Source: CAD feature listing. Evaluate the final solid. Frame: model axes, mm. Give positions to 0.01 mm unless a question says otherwise; leave off trailing zeros. Order: outer loops, then holes, each group sorted by start corner. A loop starts at its lowest first (then second) coordinate and runs counter-clockwise, first axis right, second up. Notation, with made-up numbers: M -13.5,-31 L 16.5,-31 A17 cw 16.5,-6 Z; hole C 16.25,70.25 d6. An arc over 180 degrees is marked long. Answer in a Markdown table with one row per item. Add a question column.
(1) Section query A-A, the plane z = -27. Return loops of the section in (x, y).
(2) Material intervals for line 1 along X through (y, z) = (0.7, -41); line 2 along Z through (x, y) = (-22, 1.45); line 3 along Z through (x, y) = (-28.5, 0.55) (3 decimals), sorted ascending.
(3) Section query C-C, the plane x = 22. Return loops of the section in (y, z).
(4) Section query B-B, the plane x = 34.5. Return loops of the section in (y, z).
(5) Pin query (flat end, axial travel): P1, Ø0.6, axis at x = -39.5, y = 1.5, coming from the -Z side. Return the tip coordinate at first contact, or that it passes through.
(6) Section query D-D, the plane y = 0.55. Count the separate pieces of the cut face and the enclosed holes in it, plus the area to 3 significant figures.
Autodesk Inventor part; units mm, degrees
ref_plane "YZ Plane" through (0, 0, 0) normal (1, 0, 0) x (0, 1, 0)
ref_plane "XZ Plane" through (0, 0, 0) normal (0, 1, 0) x (-1, 0, 0)
ref_plane "XY Plane" through (0, 0, 0) normal (0, 0, 1) x (1, 0, 0)
sketch "Эскиз1" plane through (0, 0, 0) normal (0, 1, 0) x (-1, 0, 0)
  circle A0 centre (0, 0) radius 55
  line L0 (0, 0) -> (0, -0.5)
  line L1 (0, 0) -> (0, 0.5)
  line L2 (1.3737, 0.5) -> (52.9976, 0.5)
  arc A1 (52.9976, 0.5) -> (40.9199, 33.6832) centre (0, 0) ccw
  arc A2 (40.2772, 34.4492) -> (9.6953, 52.1057) centre (0, 0) ccw
  arc A3 (8.7105, 52.2793) -> (-26.0658, 46.1473) centre (0, 0) ccw
  arc A4 (-26.9318, 45.6473) -> (-49.6305, 18.5961) centre (0, 0) ccw
  arc A5 (-49.9725, 17.6564) -> (-49.9725, -17.6564) centre (0, 0) ccw
  arc A6 (-49.6305, -18.5961) -> (-26.9318, -45.6473) centre (0, 0) ccw
  arc A7 (-26.0658, -46.1473) -> (8.7105, -52.2793) centre (0, 0) ccw
  arc A8 (9.6953, -52.1057) -> (40.2772, -34.4492) centre (0, 0) ccw
  arc A9 (40.9199, -33.6832) -> (52.9976, -0.5) centre (0, 0) ccw
  line L3 (-1.1199, 0.9397) -> (-49.6305, 18.5961)
  line L4 (-1.1199, 0.9397) -> (-26.9318, 45.6473)
  line L5 (-1.4619, 0) -> (-49.9725, -17.6564)
  line L6 (-1.4619, 0) -> (-49.9725, 17.6564)
  line L7 (-1.1199, -0.9397) -> (-26.9318, -45.6473)
  line L8 (0.0882, -0.5) -> (0, -0.5321)
  line L9 (-1.1199, -0.9397) -> (-49.6305, -18.5961)
  line L10 (-0.2539, -1.4397) -> (8.7105, -52.2793)
  line L11 (0.731, -1.266) -> (40.2772, -34.4492)
  line L12 (0.3889, -0.3264) -> (0.342, -0.4076)
  line L13 (-0.2539, -1.4397) -> (-26.0658, -46.1473)
  line L14 (0.731, -1.266) -> (9.6953, -52.1057)
  line L15 (0.3214, -0.383) -> (0.3889, -0.3264)
  line L16 (0.7779, 0) -> (40.9199, 33.6832)
  line L17 (0.7779, 0) -> (40.9199, -33.6832)
  line L18 (0.731, 1.266) -> (9.6953, 52.1057)
  line L19 (0.731, 1.266) -> (40.2772, 34.4492)
  line L20 (-0.2539, 1.4397) -> (-26.0658, 46.1473)
  line L21 (-0.2539, 1.4397) -> (8.7105, 52.2793)
  line L22 (0, -0.5) -> (0.0882, -0.5)
  line L23 (1.3737, -0.5) -> (52.9976, -0.5)
  dimension "d0" = 110
  dimension "d2" = 0.5
  dimension "d3" = 0.5
extrude "Выдавливание1" add sketch "Эскиз1" along normal blind 2
Values follow:
| question | item | result |
|---|---|---|
| 1 | outline | M -47.92,0 L -45.61,0 L -45.61,2 L -47.92,2 Z; M -32.96,0 L -31.4,0 L -31.4,2 L -32.96,2 Z; M -5.27,0 L -4.25,0 L -4.25,2 L -5.27,2 Z; M 15.01,0 L 16.17,0 L 16.17,2 L 15.01,2 Z; M 45.61,0 L 47.92,0 L 47.92,2 L 45.61,2 Z |
| 2 | line 1 | x = -36.66 to -33.59, -7.74 to -6.72, 23.09 to 24.25, 33.59 to 36.66 |
| 2 | line 2 | z = -50.41 to -48.22, -19.11 to -17.81, -0.5 to 0.5, 17.81 to 19.11, 48.22 to 50.41 |
| 2 | line 3 | z = -47.04 to -44.685, -24.567 to -23.262, -0.5 to 0.5, 23.262 to 24.567, 44.685 to 47.04 |
| 3 | outline | M 0,-50.41 L 2,-50.41 L 2,-48.22 L 0,-48.22 Z; M 0,-39.11 L 2,-39.11 L 2,-37.11 L 0,-37.11 Z; M 0,-8.54 L 2,-8.54 L 2,-7.48 L 0,-7.48 Z; M 0,7.48 L 2,7.48 L 2,8.54 L 0,8.54 Z; M 0,37.11 L 2,37.11 L 2,39.11 L 0,39.11 Z; M 0,48.22 L 2,48.22 L 2,50.41 L 0,50.41 Z |
| 4 | outline | M 0,-42.83 L 2,-42.83 L 2,-40.23 L 0,-40.23 Z; M 0,-13.09 L 2,-13.09 L 2,-12.02 L 0,-12.02 Z; M 0,12.02 L 2,12.02 L 2,13.09 L 0,13.09 Z; M 0,40.23 L 2,40.23 L 2,42.83 L 0,42.83 Z |
| 5 | P1 | stops at z = -38.58 |
| 6 | separate pieces | 1 |
| 6 | enclosed holes | 9 |
| 6 | area | 1,150 mm² |
